Autodesk Inventor part; units mm, degrees
ref_plane "YZ Plane" through (0, 0, 0) normal (1, 0, 0) x (0, 1, 0)
ref_plane "XZ Plane" through (0, 0, 0) normal (0, 1, 0) x (-1, 0, 0)
ref_plane "XY Plane" through (0, 0, 0) normal (0, 0, 1) x (1, 0, 0)
sketch "スケッチ1" plane through (0, 0, 0) normal (0, 0, 1) x (1, 0, 0)
  line L0 (0, 0) -> (252.35, 0)
  line L1 (252.35, 0) -> (252.35, 70)
  line L2 (252.35, 70) -> (0, 70)
  line L3 (0, 70) -> (0, 0)
  dimension "d0" = 70
  dimension "d1" = 252.35
extrude "押し出し1" add sketch "スケッチ1" along normal blind 5
sketch "スケッチ2" plane through (0, 0, 5) normal (0, 0, 1) x (1, 0, 0)
  line L0 (0, 0) -> (252.35, 0)
  line L1 (0, 70) -> (0, 0)
  point P0 (25, 35)
  dimension "d4" = 35
  dimension "d5" = 25
hole "穴1" at (25, 35, 5) direction (0, 0, -1) diameter 12 end through all
sketch "スケッチ3" plane through (0, 0, 5) normal (0, 0, 1) x (1, 0, 0)
  line L0 (252.35, 0) -> (252.35, 70)
  circle A0 centre (25, 35) radius 6
  line L1 (0, 0) -> (252.35, 0)
  point P0 (212.35, 35)
  dimension "d14" = 187.35
  dimension "d15" = 35
hole "穴2" at (212.35, 35, 5) direction (0, 0, -1) diameter 24 end through all
sketch "スケッチ4" plane through (0, 0, 5) normal (0, 0, 1) x (1, 0, 0)
  line L0 (252.35, 0) -> (252.35, 70)
  line L1 (0, 70) -> (0, 0)
  line L2 (252.35, 70) -> (0, 70)
  line L3 (0, 0) -> (252.35, 0)
  line L4 (0, 55) -> (147.35, 55)
  line L5 (0, 15) -> (147.35, 15)
  line L6 (147.35, 0) -> (147.35, 15)
  line L7 (147.35, 55) -> (147.35, 70)
  line L8 (147.35, 55) -> (0, 55)
  line L9 (0, 55) -> (0, 70)
  line L10 (0, 70) -> (147.35, 70)
  line L11 (147.35, 70) -> (147.35, 55)
  line L12 (147.35, 15) -> (0, 15)
  line L13 (0, 15) -> (0, 0)
  line L14 (0, 0) -> (147.35, 0)
  line L15 (147.35, 0) -> (147.35, 15)
  dimension "d24" = 15
  dimension "d25" = 15
extrude "押し出し2" cut sketch "スケッチ4" against normal blind 10 contours L3 L1 L5 L6 | L7 L4 L1 L2
fillet "フィレット1" radius 4 2 edges at (147.35, 15, 2.5) (147.35, 55, 2.5)
sketch "スケッチ5" plane through (0, 0, 5) normal (0, 0, 1) x (1, 0, 0)
  line L0 (147.35, 0) -> (252.35, 0)
  circle A0 centre (212.35, 35) radius 12
  point P0 (0, 0)
  point P1 (238.35, 35)
  point P2 (199.35, 57.5167)
  point P3 (199.35, 12.4833)
  dimension "d29" = 35
  dimension "d30" = 26
  dimension "d33" = 360
hole "穴3" at (238.35, 35, 5) at (199.35, 57.5167, 5) at (199.35, 12.4833, 5) direction (0, 0, -1) diameter 3.5 end through all
sketch "スケッチ6" plane through (0, 0, 5) normal (0, 0, 1) x (1, 0, 0)
  circle A0 centre (212.35, 35) radius 12
  line L0 (147.35, 0) -> (252.35, 0)
  point P0 (0, 0)
  point P1 (194.35, 35)
  point P2 (221.35, 19.4115)
  point P3 (221.35, 50.5885)
  dimension "d42" = 18
  dimension "d43" = 35
  dimension "d46" = 360
hole "穴4" at (194.35, 35, 5) at (221.35, 19.4115, 5) at (221.35, 50.5885, 5) direction (0, 0, -1) diameter 3.5 end through all
fillet "フィレット2" radius 4 6 edges at (0, 55, 2.5) (0, 15, 2.5) (147.35, 0, 2.5) (147.35, 70, 2.5) (252.35, 70, 2.5) (252.35, 0, 2.5)
sketch "スケッチ7" plane through (0, 0, 0) normal (0, 0, -1) x (-1, 0, 0)
  point P0 (0, 0)
properties part number "タイヤアーム"
Build history of the part. All positions in model axes, mm. A direction names the side the tool comes from. Round coordinates to 2 decimals unless told otherwise and drop trailing zeros. Order: outer loops, then holes, each group sorted by start corner. A loop starts at its lowest first (then second) coordinate and runs counter-clockwise, first axis right, second up. Notation, with made-up numbers: (44, 84.5) - (55, 84.5) arc R19 ccw to (55, 93.5) - close; hole circle Ø8 at (8, 74). An arc over 180 degrees is marked (long way). Use a Markdown table: item, result.
1) Saw through at B-B on z = 2.05. Give the number of separate pieces and of enclosed holes in the cut face, and give its area (3 significant figures).
Recorded:
| item | result |
|---|---|
| separate pieces | 1 |
| enclosed holes | 8 |
| area | 12,600 mm² |
2) Wall check: L1, parallel to X at y = 35, z = 2.6; L2, parallel to Y at x = 199.35, z = 2.35; L3, parallel to Y at x = 25, z = 1.65. Give the ranges that are in metal, low to high.
Recorded:
| item | result |
|---|---|
| L1 | x = 0 to 19, 31 to 192.6, 196.1 to 200.35, 224.35 to 236.6, 240.1 to 252.35 |
| L2 | y = 0 to 10.73, 14.23 to 55.77, 59.27 to 70 |
| L3 | y = 15 to 29, 41 to 55 |
3) Tool access for faces 4 (the face through (152, 35, 5)), 5 (the face through (73, 15, 3)), 6 (the face through (73, 55, 3)): list every direction of +Z, -Z, +X, -X, +Y, -Y with a clear straight run to the whole face (end or side of a thin tool).
Recorded:
| item | result |
|---|---|
| face 4 | +Z, +X, -X, +Y, -Y |
| face 5 | +Z, -Z, -X, -Y |
| face 6 | +Z, -Z, -X, +Y |
4) Pull direction X, two halves, no side cores. Call faces 1 (the face through (148.553, 1.141, 2.465)), 2 (the face through (251.209, 68.797, 2.535)), 3 (the face through (224.065, 37.601, 2.465)): pulls with the +X half, pulls with the -X half, needs draft (parallel to the pull), parting line crosses it, or undercut.
Recorded:
| item | result |
|---|---|
| face 1 | pulls with the -X half |
| face 2 | pulls with the +X half |
| face 3 | undercut |
5) Saw through at A-A on x = 212.35. Write the cut outline in (y, z), and give its area (3 significant figures).
Recorded:
| item | result |
|---|---|
| outline | (0, 0) - (23, 0) - (23, 5) - (0, 5) - close; (47, 0) - (70, 0) - (70, 5) - (47, 5) - close |
| area | 230 mm² |
6) Saw through at C-C on x = 25. Write the cut outline in (y, z), and give its area (3 significant figures).
Recorded:
| item | result |
|---|---|
| outline | (15, 0) - (29, 0) - (29, 5) - (15, 5) - close; (41, 0) - (55, 0) - (55, 5) - (41, 5) - close |
| area | 140 mm² |
7) Saw through at D-D on x = 128. Write the cut outline in (y, z).
Recorded:
| item | result |
|---|---|
| outline | (15, 0) - (55, 0) - (55, 5) - (15, 5) - close |
8) Flat gauge pins, fed straight in: pin 1 Ø1.5 at (y, z) = (46.5, 4) entering from -X; pin 2 Ø2 at (x, z) = (45, 3.5) entering from +Y; pin 3 Ø1.5 at (y, z) = (8, 3) entering from -X; pin 4 Ø1.5 at (x, z) = (93, 2.5) entering from -Y. Where does each tip first touch, or does it go through?
Recorded:
| item | result |
|---|---|
| pin 1 | stops at x = 0 |
| pin 2 | stops at y = 55 |
| pin 3 | stops at x = 147.35 |
| pin 4 | stops at y = 15 |
